from build123d import *

# Parameters (mm, degrees)
BOSS_EXTRUDE1_DEPTH                   = 63.5
F_1_4_0_25_DIAMETER_HOLE1_D           = 6.35
F_1_4_0_25_DIAMETER_HOLE1_ON_FACE_2_D = 6.35


with BuildPart() as part:
    # Sketch3 → Boss-Extrude1 (new body)
    with BuildSketch(Plane.XY):
        with BuildLine():
            Line((0, 6.35), (0, 33.655))
            ThreePointArc((0, 33.655), (-0.371974388, 34.553025612), (-1.27, 34.925))
            Line((-1.27, 34.925), (-3.175, 34.925))
            Line((-3.175, 34.925), (-3.175, 0))
            ThreePointArc((-3.175, 0), (-2.24506403, -2.24506403), (0, -3.175))
            Line((0, -3.175), (34.925, -3.175))
            Line((34.925, -3.175), (34.925, -1.27))
            ThreePointArc((34.925, -1.27), (34.553025612, -0.371974388), (33.655, 0))
            Line((33.655, 0), (6.35, 0))
            ThreePointArc((6.35, 0), (1.859871939, 1.859871939), (0, 6.35))
        make_face()
    extrude(amount=BOSS_EXTRUDE1_DEPTH)

    # 1/4 (0.25) Diameter Hole1 (through all)
    with Locations(Plane(origin=(22.225, 0, 53.975), x_dir=(1, 0, 0), z_dir=(0, 1, 0))):
        with Locations((0, 0), (0, 44.45)):
            Hole(F_1_4_0_25_DIAMETER_HOLE1_D / 2)

    # 1/4 (0.25) Diameter Hole1 on face 2 (through all)
    with Locations(Plane(origin=(0, 22.225, 9.525), x_dir=(0, 0, 1), z_dir=(1, 0, 0))):
        with Locations((0, 0), (44.45, 0)):
            Hole(F_1_4_0_25_DIAMETER_HOLE1_ON_FACE_2_D / 2)


solid = part.part
Could you check a few things on this model? Use its own coordinates, in mm. A direction names the side the tool comes from. Give positions to 0.01 mm unless a question says otherwise; leave off trailing zeros. Order: outer loops, then holes, each group sorted by start corner. A loop starts at its lowest first (then second) coordinate and runs counter-clockwise, first axis right, second up. Notation, with made-up numbers: (70.25, 8) - (100.25, 8) arc R18 ccw to (100.25, 18) - close; hole circle Ø2 at (-20, 63). An arc over 180 degrees is marked (long way). Return JSON: item names as keys, results as strings. Group by question number.
Q1. Suppose I cut it at B-B, the plane z = 35.5. Please give me the cut outline in (x, y) (3 decimals), and give its area (3 significant figures).
Q2. Will these pins go through, and if not, where does the flat tip stop? pin 1 Ø4 at (x, z) = (19.5, 12) entering from +Y; pin 2 Ø22 at (y, z) = (15, 47.5) entering from +X; pin 3 Ø22 at (x, z) = (13.5, 40.5) entering from +Y; pin 4 Ø5.5 at (x, z) = (22.225, 9.525) entering from -Y.
Q3. Suppose I cut it at C-C, the plane x = 10. Please give me the cut outline in (y, z) (3 decimals).
Q4. Suppose I cut it at A-A, the plane y = 24. Please give me the cut outline in (x, z) (3 decimals), and give its area (3 significant figures).
Q5. Thinking about a two-plate mould opening in Z: for faces 1 (the face through (19.29, -1.61, 10.74)), 2 (the face through (34.925, -2, 31)), 3 (the face through (0, 3, 63.5)), which applies, pulls with the +Z half, pulls with the -Z half, needs draft (parallel to the pull), parting line crosses it, or undercut?
Q6. Please list where this line runs through material, in increasing order: line 1 along Y through (x, z) = (16, 59) (3 decimals). Write a range as [from, to].
Q7. Which directions (+Z, -Z, +X, -X, +Y, -Y) give clear straight access to the entire face, cutting with the end or side of a thin tool? Please do faces 4 (the face through (0, 3, 0)), 5 (the face through (20, 0, 31)).
Resolved:
{
 "1": {"outline": "(-3.175, 0) arc R3.175 ccw to (0, -3.175) - (34.925, -3.175) - (34.925, -1.27) arc R1.27 ccw to (33.655, 0) - (6.35, 0) arc R6.35 cw to (0, 6.35) - (0, 33.655) arc R1.27 ccw to (-1.27, 34.925) - (-3.175, 34.925) - close", "area": "238 mm2"},
 "2": {"pin 1": "stops at y = 0", "pin 2": "stops at x = 0.45", "pin 3": "stops at y = 1.3", "pin 4": "passes through"},
 "3": {"outline": "(-3.175, 0) - (0, 0) - (0, 63.5) - (-3.175, 63.5) - close"},
 "4": {"outline": "(-3.175, 0) - (0, 0) - (0, 6.893) - (-3.175, 6.893) - close; (-3.175, 12.157) - (0, 12.157) - (0, 51.343) - (-3.175, 51.343) - close; (-3.175, 56.607) - (0, 56.607) - (0, 63.5) - (-3.175, 63.5) - close", "area": "168 mm2"},
 "5": {"face 1": "undercut", "face 2": "needs draft", "face 3": "pulls with the +Z half"},
 "6": {"line 1": "y = [-3.175, 0]"},
 "7": {"face 4": "-Z, +X, -X, +Y, -Y", "face 5": "+Z, -Z, +X, +Y"}
}
